The listing builds one solid part. Answer for the finished solid, in the listing's coordinates (mm). Coordinates: 2 decimals unless noted, no trailing zeros. Loops run counter-clockwise (first coordinate to the right, second up) from the corner with the lowest first, then second, coordinate; pieces in that order, holes last. Notation, with made-up numbers: (-40, -32) - (-26, -32) arc R12 cw to (-26, -12) - close; hole circle Ø2 at (-23.5, 27). An arc over 180 degrees is marked (long way). Return JSON: item names as keys, results as strings. Group by question number.
1. Find the intervals of material crossed by line 1 along Y through (x, z) = (696, -2.25); line 2 along Y through (x, z) = (384.5, -0.5); line 3 along X through (y, z) = (607, 2.5), in increasing order.
2. Section C-C (x = 451) is taken. Write down the section's boundary in (y, z).
3. Section B-B (y = 167.5) is taken. Write down the section's boundary in (x, z).
4. Each of these flat-tipped pins is pushed along its axis until it touches: P1, Ø5, axis at y = 439.5, z = 2.5, coming from the +X side; P2, Ø5, axis at y = 629.5, z = -3, coming from the -X side; P3, Ø4.5, axis at x = 15, y = -26, coming from the +Z side; P4, Ø5, axis at y = 192.5, z = 0, coming from the +X side. Where does it stop, or does it pass through?
5. Section A-A (z = -3.25) is taken. Write down the section's boundary in (x, y).
6. The mould has two halves that part along Y. Classify faces 1 (the face through (41.215, 23.791, 0.07)), 2 (the face through (300.71, 714.84, 0.07)), 3 (the face through (275, 673, -5)): pulls with the +Y half, pulls with the -Y half, needs draft (parallel to the pull), parting line crosses it, or undercut.
```python
from build123d import *

# Parameters (mm, degrees)
SKETCH5_R           = 3.75
BOSS_EXTRUDE1_DEPTH = 5


with BuildPart() as part:
    # Sketch5 → Boss-Extrude1 (new, symmetric)
    with BuildSketch(Plane.XY):
        with BuildLine():
            Line((1000, 980), (1000, 1000))
            ThreePointArc((1000, 1000), (292.893218813, 707.106781187), (0, 0))
            Line((0, 0), (20.017296358, 5.822418881))
            ThreePointArc((20.017296358, 5.822418881), (20.055305468, 10.411323589), (20.114802643, 15))
            Line((20.114802643, 15), (46.029376088, -17.282126934))
            ThreePointArc((46.029376088, -17.282126934), (45.913408903, -27.269346828), (36.092525555, -29.08820907))
            Line((36.092525555, -29.08820907), (18.627898207, -19.435827958))
            ThreePointArc((18.627898207, -19.435827958), (8.435827958, -22.372101793), (11.372101793, -32.564172042))
            Line((11.372101793, -32.564172042), (28.836729142, -42.216553154))
            ThreePointArc((28.836729142, -42.216553154), (55.954267895, -38.481822572), (60.055964287, -11.417358652))
            Line((60.055964287, -11.417358652), (21.838459149, 60))
            ThreePointArc((21.838459149, 60), (328.583586736, 713.862731903), (1000, 980))
        make_face()
        with Locations((15, -26)):
            Circle(SKETCH5_R, mode=Mode.SUBTRACT)
    extrude(amount=BOSS_EXTRUDE1_DEPTH, both=True)


solid = part.part
```
The answers:
{
 "1": {"line 1": "y = 931.66 to 952.67", "line 2": "y = 762.6 to 788.14", "line 3": "x = 205.3 to 230.62"},
 "2": {"outline": "(811.79, -5) - (835.82, -5) - (835.82, 5) - (811.79, 5) - close"},
 "3": {"outline": "(14.13, -5) - (34.42, -5) - (34.42, 5) - (14.13, 5) - close"},
 "4": {"P1": "stops at x = 125.34", "P2": "stops at x = 220.98", "P3": "passes through", "P4": "stops at x = 39.6"},
 "5": {"outline": "(0, 0) - (20.02, 5.82) arc R980 cw to (20.11, 15) - (46.03, -17.28) arc R7.86 cw to (36.09, -29.09) - (18.63, -19.44) arc R7.5 ccw to (11.37, -32.56) - (28.84, -42.22) arc R22.86 ccw to (60.06, -11.42) - (21.84, 60) arc R980 cw to (1000, 980) - (1000, 1000) arc R1000 ccw to start; hole circle Ø7.5 at (15, -26)"},
 "6": {"face 1": "undercut", "face 2": "pulls with the +Y half", "face 3": "needs draft"}
}
